The model under review builds one solid part; all positions refer to its coordinate system, in mm. A direction names the side the tool comes from. Round coordinates to 2 decimals unless told otherwise and drop trailing zeros. Loops run counter-clockwise (first coordinate to the right, second up) from the corner with the lowest first, then second, coordinate; pieces in that order, holes last. Notation, with made-up numbers: M -31,-37 L 25,-37 A11 cw 25,-18 Z; hole C 83,37.25 d5. An arc over 180 degrees is marked long. Answer as a JSON object with one key per item and string values. Group by question number.
Item 1: Consider section B-B (y = 5.75). Give the boundary of the cut face in (x, z).
Item 2: Consider section D-D (x = 13.5). Give the boundary of the cut face in (y, z).
Item 3: To check wall thickness, follow line 1 (X direction, y = 12, z = -12.25); line 2 (Z direction, x = 8.5, y = 0.5); line 3 (Z direction, x = 12.5, y = 7). State the ranges of each line that lie inside material, in increasing order.
Item 4: The part is to be moulded in two halves that separate along Z. For faces 5 (the face through (12, 10, -20)), 6 (the face through (8.4, 1, -4)), 7 (the face through (8.5, 1, -20.5)), say which applies: +Z half, -Z half, draft (parallel to the pull), parting line (faces both ways), or undercut.
Item 5: Tool access review of faces 1 (the face through (11, 2, -20.5)), 2 (the face through (4, 2, -9)), 3 (the face through (8.5, 17, -20.5)), 4 (the face through (16, 19, -17)): name each direction out of +Z, -Z, +X, -X, +Y, -Y from which nothing blocks a thin tool from reaching the whole face with its end or side.
Item 6: Consider section C-C (x = 9.5). State how many separate pieces and enclosed holes the cut face has, and give its area (3 significant figures).
Item 7: Insertion check: P1, Ø6.5, axis at x = 11.5, y = 8, coming from the +Z side; P2, Ø0.8, axis at x = 9, y = -0.5, coming from the +Z side; P3, Ø8, axis at x = 3, y = 7, coming from the -Z side. Each pin has a flat end and moves straight along its axis. Give the tip position at first contact, or say it passes through.
Item 8: Consider section A-A (z = -11.5). Give the boundary of the cut face in (x, y), and give its area (3 significant figures).
```python
from build123d import *

# Parameters (mm, degrees)
BASE_DEPTH        = 2
SIDES_DEPTH       = 18
NUBS_BOTTOM_DEPTH = 1
NUBS_REAR_DEPTH   = 1
SIDE_CUT_REACH    = 35.615
REAR_SLOT_DEPTH   = 34


with BuildPart() as part:
    # Base Sketch → Base (new body)
    with BuildSketch(Plane(origin=(0, 0, 0), x_dir=(1, 0, 0), z_dir=(0, 1, 0))):
        Polygon((0, 0), (2, 0), (15, 0), (17, 0), (17, 20), (0, 20), align=None)
        with BuildLine():
            Line((5.5, 13), (5.5, 7))
            ThreePointArc((5.5, 7), (8.5, 4), (11.5, 7))
            Line((11.5, 7), (11.5, 13))
            ThreePointArc((11.5, 13), (8.5, 16), (5.5, 13))
        make_face(mode=Mode.SUBTRACT)
    extrude(amount=BASE_DEPTH)

    # MainUprightSketch → Sides (add)
    with BuildSketch(Plane(origin=(0, 2, 0), x_dir=(1, 0, 0), z_dir=(0, 1, 0))):
        Polygon((17, 0), (17, 20), (0, 20), (0, 0), (2, 0), (2, 18), (15, 18), (15, 0), align=None)
    extrude(amount=SIDES_DEPTH)

    # NubsSketch → Nubs-Bottom (add)
    with BuildSketch(Plane(origin=(0, 0, 0), x_dir=(1, 0, 0), z_dir=(0, 1, 0))):
        with BuildLine():
            Line((7, 19), (10, 19))
            ThreePointArc((10, 19), (11, 18), (10, 17))
            Line((10, 17), (7, 17))
            ThreePointArc((7, 17), (6, 18), (7, 19))
        make_face()
        with BuildLine():
            Line((7, 1), (10, 1))
            ThreePointArc((10, 1), (11, 2), (10, 3))
            Line((10, 3), (7, 3))
            ThreePointArc((7, 3), (6, 2), (7, 1))
        make_face()
    extrude(amount=-NUBS_BOTTOM_DEPTH)

    # RearNubsSketch → Nubs-Rear (add)
    with BuildSketch(Plane.XY.offset(-20)):
        with BuildLine():
            Line((10, 3), (7, 3))
            ThreePointArc((7, 3), (6, 2), (7, 1))
            Line((7, 1), (10, 1))
            ThreePointArc((10, 1), (11, 2), (10, 3))
        make_face()
        with BuildLine():
            Line((10, 19), (7, 19))
            ThreePointArc((7, 19), (6, 18), (7, 17))
            Line((7, 17), (10, 17))
            ThreePointArc((10, 17), (11, 18), (10, 19))
        make_face()
    extrude(amount=-NUBS_REAR_DEPTH)

    # Cutaway Sketch → Side Cut (cut, up to next)
    with BuildSketch(Plane(origin=(0, 0, 0), x_dir=(0, 0, -1), z_dir=(1, 0, 0)), mode=Mode.PRIVATE) as side_cut_sk1:
        Polygon((0, 3), (2, 3), (17, 18), (17, 20), (0, 20), align=None)
    side_cut_tool1 = extrude(side_cut_sk1.sketch, amount=SIDE_CUT_REACH, mode=Mode.PRIVATE) & part.part
    add(side_cut_tool1.solids().sort_by_distance((0, 13.730878, -6.269122))[0], mode=Mode.SUBTRACT)
    add(side_cut_tool1.solids().sort_by_distance((0, 13.730878, -6.269122))[1], mode=Mode.SUBTRACT)

    # RearSlotSketch → Rear Slot (cut, through all)
    with BuildSketch(Plane.XY.offset(-20)):
        with BuildLine():
            Line((5.5, 13), (5.5, 7))
            ThreePointArc((5.5, 7), (8.5, 4), (11.5, 7))
            Line((11.5, 7), (11.5, 13))
            ThreePointArc((11.5, 13), (8.5, 16), (5.5, 13))
        make_face()
    extrude(amount=REAR_SLOT_DEPTH, mode=Mode.SUBTRACT)


solid = part.part
```
Geometry results:
{
 "1": {"outline": "M 0,-20 L 5.77,-20 L 5.77,-18 L 2,-18 L 2,-4.75 L 0,-4.75 Z; M 11.23,-20 L 17,-20 L 17,-4.75 L 15,-4.75 L 15,-18 L 11.23,-18 Z"},
 "2": {"outline": "M 0,-20 L 20,-20 L 20,-18 L 2,-18 L 2,0 L 0,0 Z"},
 "3": {"line 1": "x = 0 to 2, 15 to 17", "line 2": "z = -20 to -16, -4 to 0", "line 3": "z = -20 to -18"},
 "4": {"face 5": "-Z half", "face 6": "undercut", "face 7": "draft"},
 "5": {"face 1": "-Z, +X", "face 2": "+Z, +Y", "face 3": "-Z, +X, -X", "face 4": "+Z, +X, -X, +Y"},
 "6": {"separate pieces": "3", "enclosed holes": "0", "area": "37.4 mm^2"},
 "7": {"P1": "stops at z = -18", "P2": "stops at z = -1", "P3": "stops at z = -20"},
 "8": {"outline": "M 0,0 L 5.5,0 L 5.5,2 L 2,2 L 2,12.5 L 0,12.5 Z; M 11.5,0 L 17,0 L 17,12.5 L 15,12.5 L 15,2 L 11.5,2 Z", "area": "64.0 mm^2"}
}
